Part model, mm, in its own coordinate system. A direction names the side the tool comes from. Coordinates: 2 decimals unless noted, no trailing zeros. Loops run counter-clockwise (first coordinate to the right, second up) from the corner with the lowest first, then second, coordinate; pieces in that order, holes last. Notation, with made-up numbers: M 74.25,3.5 L 103.25,3.5 A22 ccw 103.25,14.5 Z; hole C 46.5,-13 d10. An arc over 180 degrees is marked long. Answer as CSV lines item,"result". Start each with the question number.
from build123d import *

# Parameters (mm, degrees)
ESBO_O1_W                = 90
ESBO_O1_H                = 70
ESBO_O1_W_2              = 82
ESBO_O1_H_2              = 62
ESBO_O1_R                = 3.5
RESSALTO_EXTRUS_O1_DEPTH = 3
ESBO_O1_3_W              = 90
ESBO_O1_3_H              = 70
ESBO_O1_3_W_2            = 82
ESBO_O1_3_H_2            = 62
RESSALTO_EXTRUS_O2_DEPTH = 30
FILETE1_R                = 3
CORTE_EXTRUS_O1_REACH    = 103.119
FILETE2_R                = 5


with BuildPart() as part:
    # Esbo_o1 → Ressalto-extrus_o1 (new body)
    # profile 1 of 2: a face of its own
    with BuildSketch(Plane(origin=(0, 0, 0), x_dir=(1, 0, 0), z_dir=(0, 1, 0))):
        Rectangle(ESBO_O1_W, ESBO_O1_H)
        Rectangle(ESBO_O1_W_2, ESBO_O1_H_2, mode=Mode.SUBTRACT)
    # profile 2 of 2: a face of its own
    with BuildSketch(Plane(origin=(0, 0, 0), x_dir=(1, 0, 0), z_dir=(0, 1, 0))):
        Rectangle(ESBO_O1_W_2, ESBO_O1_H_2)
        with Locations(Location((0, 0, 0), (0, 0, 270))):
            Circle(ESBO_O1_R, mode=Mode.SUBTRACT)
    extrude(amount=RESSALTO_EXTRUS_O1_DEPTH)

    # Esbo_o1_3 → Ressalto-extrus_o2 (add)
    with BuildSketch(Plane(origin=(0, 0, 0), x_dir=(1, 0, 0), z_dir=(0, 1, 0))):
        Rectangle(ESBO_O1_3_W, ESBO_O1_3_H)
        Rectangle(ESBO_O1_3_W_2, ESBO_O1_3_H_2, mode=Mode.SUBTRACT)
    extrude(amount=RESSALTO_EXTRUS_O2_DEPTH)

    # Filete1
    filete1_edges = [part.edges().sort_by_distance(p)[0] for p in [
        (45, 15, 35),
        (-45, 15, 35),
        (-45, 15, -35),
        (45, 15, -35),
        (0, 0, 35),
        (-45, 0, 0),
        (0, 0, -35),
        (45, 0, 0),
    ]]
    fillet(filete1_edges, radius=FILETE1_R)

    # Esbo_o2 → Corte-extrus_o1 (cut, up to next)
    with BuildSketch(Plane(origin=(45, 0, 0), x_dir=(0, 0, -1), z_dir=(1, 0, 0)), mode=Mode.PRIVATE) as corte_extrus_o1_sk1:
        with BuildLine():
            Line((-2.5, 27.5), (-2.5, 30))
            Line((-2.5, 30), (2.5, 30))
            Line((2.5, 30), (2.5, 27.5))
            ThreePointArc((2.5, 27.5), (0, 25), (-2.5, 27.5))
        make_face()
    corte_extrus_o1_tool1 = extrude(corte_extrus_o1_sk1.sketch, amount=-CORTE_EXTRUS_O1_REACH, mode=Mode.PRIVATE) & part.part
    add(corte_extrus_o1_tool1.solids().sort_by_distance((45, 27.733375, 0))[0], mode=Mode.SUBTRACT)

    # Filete2
    filete2_edges = [part.edges().sort_by_distance(p)[0] for p in [
        (-41, 16.5, 31),
        (-41, 16.5, -31),
        (41, 16.5, -31),
        (41, 16.5, 31),
    ]]
    fillet(filete2_edges, radius=FILETE2_R)


solid = part.part
Q1. Slice it at A-A, the plane z = 0. Write the cut outline in (x, y), and give its area (3 significant figures).
Q2. Slice it at D-D, the plane z = -24. Write the cut outline in (x, y).
Q3. Two-plate mould, pull along X, no slides. Class faces 1 (the face through (-45, 16, 0)), 2 (the face through (-39, 17, 30)), 3 (the face through (44.1, 0.86, -0.45)): +X half, -X half, draft (parallel to the pull), parting line (faces both ways), or undercut.
Q4. Wall check: L1, parallel to Z at x = -2.5, y = 25.5; L2, parallel to X at y = 21.5, z = 22; L3, parallel to Y at x = 40.5, z = -10. Give the ranges that are in metal, low to high.
Q5. Slice it at B-B, the plane x = -24. Write the cut outline in (y, z).
Q6. Tool access for faces 4 (the face through (43, 25, 0)), 5 (the face through (-3.417, 1.479, -0.759)), 6 (the face through (-40, 17, -29)): list every direction of +Z, -Z, +X, -X, +Y, -Y with a clear straight run to the whole face (end or side of a thin tool).
Q7. Slice it at C-C, the plane y = 22. Write the cut outline in (x, z).
Q8. Flat gauge pin, fed straight in: P1, Ø6, axis at x = -29.5, z = 5, coming from the +Y side. Where does the tip first touch, or does it go through?
Solved:
1,outline,"M -45,3 A3 ccw -42,0 L -3.5,0 L -3.5,3 L -41,3 L -41,30 L -45,30 Z; M 3.5,0 L 42,0 A3 ccw 45,3 L 45,25 L 41,25 L 41,3 L 3.5,3 Z"
1,area,"441 mm2"
2,outline,"M -45,3 A3 ccw -42,0 L 42,0 A3 ccw 45,3 L 45,30 L 41,30 L 41,3 L -41,3 L -41,30 L -45,30 Z"
3,face 1,"-X half"
3,face 2,"undercut"
3,face 3,"+X half"
4,L1,"z = -35 to -31, 31 to 35"
4,L2,"x = -45 to -41, 41 to 45"
4,L3,"y = 0 to 3"
5,outline,"M 0,-32 A3 ccw 3,-35 L 30,-35 L 30,-31 L 3,-31 L 3,31 L 30,31 L 30,35 L 3,35 A3 ccw 0,32 Z"
6,face 4,"+X, +Y"
6,face 5,"+Y, -Y"
6,face 6,"+Y"
7,outline,"M -45,-32 A3 ccw -42,-35 L 42,-35 A3 ccw 45,-32 L 45,32 A3 ccw 42,35 L -42,35 A3 ccw -45,32 Z; hole M -41,-26 A5 ccw -36,-31 L 36,-31 A5 ccw 41,-26 L 41,26 A5 ccw 36,31 L -36,31 A5 ccw -41,26 Z"
8,P1,"stops at y = 3"
